from build123d import *

# Parameters (mm, degrees)
SKETCH1_W               = 8
SKETCH1_H               = 5
SKETCH1_H_2             = 52.6
BOSS_EXTRUDE1_DEPTH     = 10
SKETCH2_R               = 1.7
CUT_EXTRUDE1_DEPTH      = 55.870392745
CUT_EXTRUDE2_DEPTH      = 40
CUT_EXTRUDE2_DEPTH_BACK = 2.5
SKETCH3_R               = 2.85
FILLET1_DEPTH           = 2.1499999
FILLET1_START           = 7.8500001
FILLET1_2_DEPTH         = 2.1499999
FILLET1_START_2         = 0.9438
FILLET1_3_DEPTH         = 2.356451924
FILLET1_START_3         = 6.7000001
FILLET1_4_DEPTH         = 2.2437999
FILLET1_START_4         = 2.1499999
FILLET1_5_DEPTH         = 5.7000002
FILLET1_6_OUTLINE_W     = 1.7
FILLET1_6_OUTLINE_H     = 2.386959423
FILLET1_6_OUTLINE_W_2   = 2.85
FILLET1_6_OUTLINE_H_2   = 3.868292879
FILLET2_R               = 1


with BuildPart() as part:
    # Sketch1 → Boss-Extrude1 (new body)
    with BuildSketch(Plane.XY):
        with Locations((-8, 23.8)):
            Rectangle(SKETCH1_W, SKETCH1_H)
        Rectangle(SKETCH1_W, SKETCH1_H_2)
        with Locations((-8, -23.8)):
            Rectangle(SKETCH1_W, SKETCH1_H)
    extrude(amount=BOSS_EXTRUDE1_DEPTH)

    # Sketch2 → Cut-Extrude1 (cut, through all)
    with BuildSketch(Plane(origin=(0, 26.3, 0), x_dir=(1, 0, 0), z_dir=(0, 1, 0))):
        with Locations(Location((-8, -5, 0), (0, 0, 270))):
            Circle(SKETCH2_R)
    extrude(amount=-CUT_EXTRUDE1_DEPTH, mode=Mode.SUBTRACT)

    # Sketch3 → Cut-Extrude2 (cut, two sides: drawn at the far end of the back side and taken through both)
    with BuildSketch(Plane(origin=(0, -21.3, 0), x_dir=(1, 0, 0), z_dir=(0, 1, 0)).offset(-CUT_EXTRUDE2_DEPTH_BACK)):
        with Locations((-8, -5)):
            Circle(SKETCH3_R)
    extrude(amount=CUT_EXTRUDE2_DEPTH + CUT_EXTRUDE2_DEPTH_BACK, mode=Mode.SUBTRACT)

    # Fillet1: read off the stored shape, not the designer's step
    # Fillet1 outline → Fillet1 (add)
    with BuildSketch(Plane.XY):
        with BuildLine():
            ThreePointArc((-12, 21.3), (-6.343145751, 18.956854249), (-4, 13.3))
            Line((-4, 13.3), (-4, 21.3))
            Line((-4, 21.3), (-12, 21.3))
        make_face()
        with BuildLine():
            Line((-4, -21.3), (-4, -13.3))
            ThreePointArc((-4, -13.3), (-6.343145751, -18.956854249), (-12, -21.3))
            Line((-12, -21.3), (-4, -21.3))
        make_face()
    extrude(amount=FILLET1_DEPTH)

    # Fillet1 2 outline → Fillet1 2 (add)
    with BuildSketch(Plane.XY.offset(FILLET1_START)):
        with BuildLine():
            ThreePointArc((-12, 21.3), (-6.343145751, 18.956854249), (-4, 13.3))
            Line((-4, 13.3), (-4, 21.3))
            Line((-4, 21.3), (-12, 21.3))
        make_face()
        with BuildLine():
            Line((-4, -21.3), (-4, -13.3))
            ThreePointArc((-4, -13.3), (-6.343145751, -18.956854249), (-12, -21.3))
            Line((-12, -21.3), (-4, -21.3))
        make_face()
    extrude(amount=FILLET1_2_DEPTH)

    # Fillet1 3 outline → Fillet1 3 (add)
    with BuildSketch(Plane.XY.offset(FILLET1_START_2)):
        with BuildLine():
            ThreePointArc((-12, 21.3), (-6.343145751, 18.956854249), (-4, 13.3))
            Line((-4, 13.3), (-4, 21.3))
            Line((-4, 21.3), (-12, 21.3))
        make_face()
    extrude(amount=FILLET1_3_DEPTH)

    # Fillet1 4 outline → Fillet1 4 (add)
    with BuildSketch(Plane.XY.offset(FILLET1_START_3)):
        with BuildLine():
            ThreePointArc((-12, 21.3), (-6.343145751, 18.956854249), (-4, 13.3))
            Line((-4, 13.3), (-4, 21.3))
            Line((-4, 21.3), (-12, 21.3))
        make_face()
    extrude(amount=FILLET1_4_DEPTH)

    # Fillet1 5 outline → Fillet1 5 (add)
    with BuildSketch(Plane.XY.offset(FILLET1_START_4)):
        with BuildLine():
            ThreePointArc((-12, 21.3), (-6.343145751, 18.956854249), (-4, 13.3))
            Line((-4, 13.3), (-4, 21.3))
            Line((-4, 21.3), (-12, 21.3))
        make_face()
        with BuildLine():
            Line((-4, -21.3), (-4, -13.3))
            ThreePointArc((-4, -13.3), (-6.343145751, -18.956854249), (-12, -21.3))
            Line((-12, -21.3), (-4, -21.3))
        make_face()
    extrude(amount=FILLET1_5_DEPTH)

    # Fillet1 6 outline → Fillet1 6 (revolve, cut)
    with BuildSketch(Plane(origin=(-8, 0, 5), x_dir=(1, 0, 0), z_dir=(0, 0, 1))):
        with Locations((0.85, 20.106520289)):
            Rectangle(FILLET1_6_OUTLINE_W, FILLET1_6_OUTLINE_H)
        with Locations((1.425, -19.36585356)):
            Rectangle(FILLET1_6_OUTLINE_W_2, FILLET1_6_OUTLINE_H_2)
    revolve(axis=Axis((-8, 0, 5), (0, 1, 0)), mode=Mode.SUBTRACT)

    # Fillet2
    fillet2_edges = [part.edges().sort_by_distance(p)[0] for p in [
        (4, 0, 0),
        (-4, -26.3, 0),
        (-12, -23.8, 0),
        (-12, 23.8, 10),
        (-12, 23.8, 0),
        (-4, 26.3, 0),
        (4, 26.3, 5),
        (4, -26.3, 5),
        (-12, -26.3, 5),
        (-12, -21.3, 5),
        (-12, 21.3, 5),
        (-12, 26.3, 5),
        (-12, -23.8, 10),
        (-4, -26.3, 10),
        (4, 0, 10),
        (-4, 0, 0),
        (-4, 0, 10),
        (-6.343145751, 18.956854249, 0),
        (-4, 26.3, 10),
        (-6.343145751, 18.956854249, 10),
        (-6.343145751, -18.956854249, 0),
        (-6.343145751, -18.956854249, 10),
    ]]
    fillet(fillet2_edges, radius=FILLET2_R)


solid = part.part
Geometry: final body of the model. Coordinates: model frame, mm. A direction names the side the tool comes from. Coordinates: 2 decimals unless noted, no trailing zeros. Loops run counter-clockwise (first coordinate to the right, second up) from the corner with the lowest first, then second, coordinate; pieces in that order, holes last. Notation, with made-up numbers: (32, 21.5) - (84, 21.5) arc R17 cw to (84, 54.5) - close; hole circle Ø10 at (28, -26). An arc over 180 degrees is marked (long way). Put each result on its own line as item: value. Start each with the question number.
Q1. Cut plane A-A, the plane y = -23. Return loops of the section in (x, z), and give its area (3 significant figures).
Q2. Line query: line 1 (X direction, y = -24.55, z = 5); line 2 (X direction, y = 22, z = 4.5); line 3 (Z direction, x = -7, y = 22). Output: solid intervals per line, ascending.
Q3. Pull-direction query (Y, two-part tool) for faces 1 (the cylindrical face through (-3.902, -26.015, 0.301)), 2 (the flat face through (-4, 0, 5)), 3 (the flat face through (-12, 24, 5)), 4 (the flat face through (-4, 26.3, 5)); classes: released by +Y, released by -Y, zero draft, split by the parting line, or undercut.
Q4. Pin query (flat end, axial travel): pin 1 Ø2.5 at (x, z) = (-8, 5) entering from +Y; pin 2 Ø1 at (y, z) = (11.5, 6.5) entering from -X. Return the tip coordinate at first contact, or that it passes through.
Q5. Set-up query: faces 5 (the cylindrical face through (-4.098, 26.015, 9.699)), 6 (the flat face through (-8, -23.8, 7)), 7 (the cylindrical face through (-6.1, 18.7, 4.9)). Return all of +Z, -Z, +X, -X, +Y, -Y with unobstructed straight access to the full face (end or side cutting, diameter ignored); none if empty.
Q6. Cut plane D-D, the plane y = 4. Return loops of the section in (x, z), and give its area (3 significant figures).
Q7. Cut plane C-C, the plane z = 4. Return loops of the section in (x, y).
Filled sheet:
1. outline: (-12, 1) arc R1 ccw to (-11, 0) - (3, 0) arc R1 ccw to (4, 1) - (4, 9) arc R1 ccw to (3, 10) - (-11, 10) arc R1 ccw to (-12, 9) - close; hole circle Ø5.7 at (-8, 5)
1. area: 134 mm²
2. line 1: -12 to -9.7, -6.3 to 4
2. line 2: -11.97 to -9.62, -6.38 to 4
2. line 3: 0 to 3.63, 6.37 to 10
3. face 1: released by -Y
3. face 2: undercut
3. face 3: zero draft
3. face 4: released by +Y
4. pin 1: through
4. pin 2: x = -4
5. face 5: +Z, +X, -X, +Y
5. face 6: none
5. face 7: +Z, -Z, -X
6. outline: (-4, 1) arc R1 ccw to (-3, 0) - (3, 0) arc R1 ccw to (4, 1) - (4, 9) arc R1 ccw to (3, 10) - (-3, 10) arc R1 ccw to (-4, 9) - close
6. area: 79.1 mm²
7. outline: (-12, -25.3) arc R1 ccw to (-11, -26.3) - (-9.37, -26.3) - (-9.37, -23.8) - (-10.67, -23.8) - (-10.67, -21.19) arc R8 cw to (-11.11, -21.25) arc R1 ccw to (-12, -22.24) - close; (-12, 22.24) arc R1 ccw to (-11.11, 21.25) arc R8 cw to (-9.37, 20.86) - (-9.37, 26.3) - (-11, 26.3) arc R1 ccw to (-12, 25.3) - close; (-6.63, -26.3) - (3, -26.3) arc R1 ccw to (4, -25.3) - (4, 25.3) arc R1 ccw to (3, 26.3) - (-6.63, 26.3) - (-6.63, 19.23) arc R8 cw to (-4, 13.3) - (-4, -13.3) arc R8 cw to (-5.33, -17.72) - (-5.33, -23.8) - (-6.63, -23.8) - close
